from build123d import *

# Parameters (mm, degrees)
ESQUISSE1_R             = 2.1
BOSS_EXTRU_1_DEPTH      = 3
ESQUISSE2_R             = 2.1
ENL_V_MAT_EXTRU_1_DEPTH = 166.707573756


with BuildPart() as part:
    # Esquisse1 → Boss.-Extru.1 (new body)
    with BuildSketch(Plane.XY):
        with BuildLine():
            Line((0, 15), (150, 15))
            ThreePointArc((150, 15), (165, 0), (150, -15))
            Line((150, -15), (0, -15))
            Line((0, -15), (0, 15))
        make_face()
        with Locations((150, 0)):
            Circle(ESQUISSE1_R, mode=Mode.SUBTRACT)
    extrude(amount=BOSS_EXTRU_1_DEPTH)

    # Symétrie1: part across plane


with BuildPart() as part_1:
    add(part.part)
    add(part.part.mirror(Plane(origin=(0, 15, 3), x_dir=(0, 0, 1), z_dir=(1, 0, 0))))

    # Esquisse2 → Enlèv. mat.-Extru.1 (cut, through all)
    with BuildSketch(Plane.XY.offset(3)):
        with Locations((-80, 0)):
            Circle(ESQUISSE2_R)
    extrude(amount=-ENL_V_MAT_EXTRU_1_DEPTH, mode=Mode.SUBTRACT)


solid = part_1.part
CAD build for the part. Positions are in the model's coordinates, mm. Round coordinates to 2 decimals unless told otherwise and drop trailing zeros. Loops run counter-clockwise (first coordinate to the right, second up) from the corner with the lowest first, then second, coordinate; pieces in that order, holes last.
(1) Cut at A-A (z = 1.2). Give the cut face in (x, y).
(2) Drop flat-ended pins along their axis: pin 1 (3.5 mm diameter, centred on x = 150, y = 0, fed in from +Z); pin 2 (1 mm diameter, centred on y = 8, z = 2.5, fed in from -X). Give the stop position or say it passes through.
(3) Cut at B-B (y = 9.5). Give the cut face in (x, z), plus the area to 3 significant figures.
(4) Wall check: line 1 along Y through (x, z) = (-80, 1.7); line 2 along X through (y, z) = (0.75, 1.5); line 3 along X through (y, z) = (1.25, 2.75). Give the ranges that are in metal, low to high.
Findings below:
1. outline: (-150, -15) - (150, -15) arc R15 ccw to (150, 15) - (-150, 15) arc R15 ccw to start; hole circle Ø4.2 at (-150, 0); hole circle Ø4.2 at (-80, 0); hole circle Ø4.2 at (150, 0)
2. pin 1: passes through
2. pin 2: stops at x = -162.99
3. outline: (-161.61, 0) - (161.61, 0) - (161.61, 3) - (-161.61, 3) - close
3. area: 970 mm2
4. line 1: y = -15 to -2.1, 2.1 to 15
4. line 2: x = -164.98 to -151.96, -148.04 to -81.96, -78.04 to 148.04, 151.96 to 164.98
4. line 3: x = -164.95 to -151.69, -148.31 to -81.69, -78.31 to 148.31, 151.69 to 164.95
